Check sheet for the modelled part. Datum: model origin and axes. Units: mm. A direction names the side the tool comes from. Give positions to 0.01 mm unless a question says otherwise; leave off trailing zeros. Loops run counter-clockwise (first coordinate to the right, second up) from the corner with the lowest first, then second, coordinate; pieces in that order, holes last. Notation, with made-up numbers: (-23, 24) -> (12, 24) arc R22 ccw to (12, 35) -> close; hole circle Ø9 at (5.5, -1.75). An arc over 180 degrees is marked (long way). Write each question's results on one line, items separated by ' | '. Start each with the question number.
1. Material ranges on L1, parallel to Z at x = -37, y = -12; L2, parallel to X at y = 41, z = 18.5; L3, parallel to Y at x = -26, z = 1, recorded low to high. Write a range as from..to.
2. Cross-section at C-C on z = 24.5. Record the boundary of the cut face in (x, y).
3. Cross-section at B-B on x = -1. Record the boundary of the cut face in (y, z).
4. Mould release check, pull along Y, two halves, no side actions. Record for faces 4 (the face through (-1, 0, 0)), 5 (the face through (40.878, -16.827, 1.479)), 6 (the face through (-1, -20, 1)): +Y half, -Y half, draft (parallel to the pull), parting line (faces both ways), or undercut.
5. Cross-section at A-A on y = 46.5. Record the boundary of the cut face in (x, z).
6. Cross-section at D-D on y = 22.5. Record the boundary of the cut face in (x, z), and give its area (3 significant figures).
7. Gauge pin test, flat ends, axial feed: pin 1 Ø2.5 at (y, z) = (36.5, 2) entering from +X; pin 2 Ø3.5 at (x, z) = (-46.5, 1.5) entering from +Y; pin 3 Ø1.5 at (y, z) = (38.5, 24.5) entering from -X. Record the tip position at first contact, or that the pin passes through.
8. Tool access check on faces 1 (the face through (35, 20, 1)), 2 (the face through (-8.2, 50, 7.7)), 3 (the face through (5, 20, 2)). Record the directions out of +Z, -Z, +X, -X, +Y, -Y that give a thin tool (end or side, any length) a straight path to the whole face; none if there is none.
from build123d import *

# Parameters (mm, degrees)
EXTRUDE_1_DEPTH     = 3
SKETCH_2_W          = 2
SKETCH_2_H          = 30
EXTRUDE_2_DEPTH     = 25
CUT_EXTRUDE_1_REACH = 84.006
SKETCH_5_W          = 10
SKETCH_5_H          = 14.402378288
HOLE_WIZARD_M3_2_D  = 2.5
HOLE_WIZARD_M3_3_D  = 2.5


with BuildPart() as part:
    # 草图1 → 凸台-拉伸1 (new body)
    with BuildSketch(Plane.XY):
        Polygon((-60, 20), (-60, -20), (60, -20), (60, 20), (10, 20), (10, 50), (-10, 50), (-10, 20), align=None)
    extrude(amount=EXTRUDE_1_DEPTH)

    # 草图2 → 凸台-拉伸2 (add)
    with BuildSketch(Plane.XY.offset(3)):
        with Locations((-9, 35)):
            Rectangle(SKETCH_2_W, SKETCH_2_H)
    extrude(amount=EXTRUDE_2_DEPTH)

    # 草图5 → 切除-拉伸1 (cut, up to next)
    with BuildSketch(Plane.XY.offset(3), mode=Mode.PRIVATE) as cut_extrude_1_sk1:
        with Locations((0, 20.369307695)):
            Rectangle(SKETCH_5_W, SKETCH_5_H)
    cut_extrude_1_tool1 = extrude(cut_extrude_1_sk1.sketch, amount=-CUT_EXTRUDE_1_REACH, mode=Mode.PRIVATE) & part.part
    add(cut_extrude_1_tool1.solids().sort_by_distance((0, 20.369308, 3))[0], mode=Mode.SUBTRACT)

    # M3 螺纹孔2 (through all)
    with Locations(Plane.ZY.offset(10)):
        with Locations((24.5, 46.5), (24.5, 22.5)):
            Hole(HOLE_WIZARD_M3_2_D / 2)

    # M3 螺纹孔3 (through all)
    with Locations(Plane.XY.offset(3)):
        with Locations((-40.606601718, 5.606601718), (-19.393398282, 5.606601718), (-19.393398282, -15.606601718), (-40.606601718, -15.606601718), (19.393398282, 5.606601718), (40.606601718, 5.606601718), (19.393398282, -15.606601718), (40.606601718, -15.606601718)):
            Hole(HOLE_WIZARD_M3_3_D / 2)


solid = part.part
Geometry says:
1) L1: 0..3 | L2: -10..-8 | L3: -20..20
2) outline: (-10, 20) -> (-8, 20) -> (-8, 21.25) -> (-10, 21.25) -> close; (-10, 23.75) -> (-8, 23.75) -> (-8, 45.25) -> (-10, 45.25) -> close; (-10, 47.75) -> (-8, 47.75) -> (-8, 50) -> (-10, 50) -> close
3) outline: (-20, 0) -> (13.17, 0) -> (13.17, 3) -> (-20, 3) -> close; (27.57, 0) -> (50, 0) -> (50, 3) -> (27.57, 3) -> close
4) face 4: draft | face 5: undercut | face 6: -Y half
5) outline: (-10, 0) -> (10, 0) -> (10, 3) -> (-8, 3) -> (-8, 23.25) -> (-10, 23.25) -> close; (-10, 25.75) -> (-8, 25.75) -> (-8, 28) -> (-10, 28) -> close
6) outline: (-10, 0) -> (-5, 0) -> (-5, 3) -> (-8, 3) -> (-8, 23.25) -> (-10, 23.25) -> close; (-10, 25.75) -> (-8, 25.75) -> (-8, 28) -> (-10, 28) -> close; (5, 0) -> (10, 0) -> (10, 3) -> (5, 3) -> close | area: 75.0 mm^2
7) pin 1: x = 10 | pin 2: y = 20 | pin 3: x = -10
8) face 1: +Z, -Z, +X, +Y | face 2: +Z, -Z, +X, -X, +Y | face 3: +Z, -Z
